Verification items for the finished model (mm, model axes). A direction names the side the tool comes from. Round coordinates to 2 decimals unless told otherwise and drop trailing zeros. Loops run counter-clockwise (first coordinate to the right, second up) from the corner with the lowest first, then second, coordinate; pieces in that order, holes last. Notation, with made-up numbers: (-30, 81) - (11, 81) arc R17 cw to (11, 89) - close; hole circle Ø1 at (52, 51.5). An arc over 180 degrees is marked (long way). Use a Markdown table: item, result. Add a question column.
```python
from build123d import *

# Parameters (mm, degrees)
SCHNITT_LINEAR_AUSTRAGEN1_DEPTH = 20.697715604


with BuildPart() as part:
    # Skizze1 → Rotation1 (revolve)
    with BuildSketch(Plane.XY, mode=Mode.PRIVATE) as rotation1_sk:
        Polygon((0, 0), (0, 7), (2.9, 7), (2.9, 9.925), (7.1, 9.925), (7.1, 12), (10, 12), (10, 0), align=None)
    revolve(rotation1_sk.sketch.rotate(Axis((0, 0, 0), (-1, 0, 0)), 90), axis=Axis((0, 0, 0), (-1, 0, 0)))

    # Skizze2 → Schnitt-Linear austragen1 (cut, through all)
    with BuildSketch(Plane.ZY):
        with BuildLine():
            Line((-2.75, 3.04097024), (2.75, 3.04097024))
            ThreePointArc((2.75, 3.04097024), (0, -4.1), (-2.75, 3.04097024))
        make_face()
    extrude(amount=-SCHNITT_LINEAR_AUSTRAGEN1_DEPTH, mode=Mode.SUBTRACT)


solid = part.part
```
Q1. Set-up check for faces 4 (the face through (0, 3.01, 3.01)), 5 (the face through (2.9, -7, 2)), 6 (the face through (5, 3.041, 0)): record each of +Z, -Z, +X, -X, +Y, -Y from which the full face is reachable in a straight line by a thin tool's end or side.
Q2. Section check A-A on z = 0. Record the cut outline in (x, y) (3 decimals).
Q3. Thickness scan on line 1 along Y through (x, z) = (5.75, 0) (3 decimals); line 2 along Y through (x, z) = (7.5, 0); line 3 along X through (y, z) = (-9, 2.5). Record the ranges inside material, lowest first.
Q4. Section check C-C on x = 9. Record the cut outline in (y, z), plus the area to 3 significant figures.
Q5. Section check D-D on y = -7.5. Record the cut outline in (x, z).
Q6. Section check B-B on y = 0. Record the cut outline in (x, z) (3 decimals).
Q7. Go/stop test with flat-tipped pins: pin 1 Ø9.5 at (y, z) = (0, 0) entering from +X; pin 2 Ø6 at (x, z) = (4.5, 7) entering from +Y; pin 3 Ø2 at (x, z) = (5.5, 9) entering from -Y; pin 4 Ø4 at (x, z) = (5, -4.5) entering from -Y (3 decimals). Record where each tip stops, or that it passes through.
Q8. Release check for a two-part mould opening along Y. For faces 1 (the face through (5.029, 6.039, 7.876)), 2 (the face through (10, 0, -5)), 3 (the face through (4.9, -4.1, 0.1)) record: +Y half, -Y half, draft (parallel to the pull), parting line (faces both ways), or undercut.
Determined:
| question | item | result |
|---|---|---|
| 1 | face 4 | +Z, -Z, -X, +Y, -Y |
| 1 | face 5 | -X |
| 1 | face 6 | +X, -X |
| 2 | outline | (0, -7) - (2.9, -7) - (2.9, -9.925) - (7.1, -9.925) - (7.1, -12) - (10, -12) - (10, -4.1) - (0, -4.1) - close; (0, 3.041) - (10, 3.041) - (10, 12) - (7.1, 12) - (7.1, 9.925) - (2.9, 9.925) - (2.9, 7) - (0, 7) - close |
| 3 | line 1 | y = -9.925 to -4.1, 3.041 to 9.925 |
| 3 | line 2 | y = -12 to -4.1, 3.04 to 12 |
| 3 | line 3 | x = 2.9 to 10 |
| 4 | outline | circle Ø24 at (0, 0); hole (3.04, -2.75) - (3.04, 2.75) arc R4.1 ccw (long way) to start |
| 4 | area | 404 mm² |
| 5 | outline | (2.9, -6.5) - (7.1, -6.5) - (7.1, -9.37) - (10, -9.37) - (10, 9.37) - (7.1, 9.37) - (7.1, 6.5) - (2.9, 6.5) - close |
| 6 | outline | (0, -7) - (2.9, -7) - (2.9, -9.925) - (7.1, -9.925) - (7.1, -12) - (10, -12) - (10, -4.1) - (0, -4.1) - close; (0, 4.1) - (10, 4.1) - (10, 12) - (7.1, 12) - (7.1, 9.925) - (2.9, 9.925) - (2.9, 7) - (0, 7) - close |
| 7 | pin 1 | stops at x = 10 |
| 7 | pin 2 | stops at y = 10.66 |
| 7 | pin 3 | stops at y = -5.87 |
| 7 | pin 4 | stops at y = -9.605 |
| 8 | face 1 | parting line |
| 8 | face 2 | draft |
| 8 | face 3 | undercut |
